from build123d import *

# Parameters (mm, degrees)
F1_DEPTH = 12


with BuildPart() as f1:
    # F0 (on Top) → F1 (new body)
    with BuildSketch(Plane.XY):
        Polygon((395, 100), (0, 100), (-395, 100), (-395, -100), (0, -100), (395, -100), align=None)
        with BuildLine():
            Line((-285.5, 60), (-243.5, 60))
            ThreePointArc((-243.5, 60), (-239.257359, 58.242641), (-237.5, 54))
            Line((-237.5, 54), (-237.5, -54))
            ThreePointArc((-237.5, -54), (-239.257359, -58.242641), (-243.5, -60))
            Line((-243.5, -60), (-285.5, -60))
            ThreePointArc((-285.5, -60), (-289.742641, -58.242641), (-291.5, -54))
            Line((-291.5, -54), (-291.5, 54))
            ThreePointArc((-291.5, 54), (-289.742641, 58.242641), (-285.5, 60))
        make_face(mode=Mode.SUBTRACT)
        with BuildLine():
            ThreePointArc((237.5, 54), (239.257359, 58.242641), (243.5, 60))
            Line((243.5, 60), (285.5, 60))
            ThreePointArc((285.5, 60), (289.742641, 58.242641), (291.5, 54))
            Line((291.5, 54), (291.5, -54))
            ThreePointArc((291.5, -54), (289.742641, -58.242641), (285.5, -60))
            Line((285.5, -60), (243.5, -60))
            ThreePointArc((243.5, -60), (239.257359, -58.242641), (237.5, -54))
            Line((237.5, -54), (237.5, 54))
        make_face(mode=Mode.SUBTRACT)
    extrude(amount=F1_DEPTH)


solid = f1.part
Can you work these out from the model? Positions are in its coordinate system, mm. Round coordinates to 2 decimals unless told otherwise and drop trailing zeros. Write each loop counter-clockwise with the first axis right and the second up, starting at its lowest first coordinate (ties: lowest second). Pieces come first, ordered by that corner, then holes. Notation, with made-up numbers: (-15.75, -12) - (43.25, -12) arc R6 cw to (43.25, -7) - close; hole circle Ø6 at (66, 11). An arc over 180 degrees is marked (long way). Write each question's results on one line, items separated by ' | '. Start each with the question number.
1) Suppose I cut it at C-C (z = 2.5). List the corners of the cut face in (x, y) for me.
2) Please list where these lines run through material, in increasing order: line 1 (X direction, y = 28, z = 2.25); line 2 (Y direction, x = -274.5, z = 4.75); line 3 (X direction, y = -57, z = 6).
3) Suppose I cut it at A-A (x = 267.5). List the corners of the cut face in (y, z) for me, and give its area (3 significant figures).
4) Suppose I cut it at B-B (y = 32.5). List the corners of the cut face in (x, z) for me.
Here are the results:
1) outline: (-395, -100) - (395, -100) - (395, 100) - (-395, 100) - close; hole (-291.5, -54) arc R6 ccw to (-285.5, -60) - (-243.5, -60) arc R6 ccw to (-237.5, -54) - (-237.5, 54) arc R6 ccw to (-243.5, 60) - (-285.5, 60) arc R6 ccw to (-291.5, 54) - close; hole (237.5, -54) arc R6 ccw to (243.5, -60) - (285.5, -60) arc R6 ccw to (291.5, -54) - (291.5, 54) arc R6 ccw to (285.5, 60) - (243.5, 60) arc R6 ccw to (237.5, 54) - close
2) line 1: x = -395 to -291.5, -237.5 to 237.5, 291.5 to 395 | line 2: y = -100 to -60, 60 to 100 | line 3: x = -395 to -290.7, -238.3 to 238.3, 290.7 to 395
3) outline: (-100, 0) - (-60, 0) - (-60, 12) - (-100, 12) - close; (60, 0) - (100, 0) - (100, 12) - (60, 12) - close | area: 960 mm2
4) outline: (-395, 0) - (-291.5, 0) - (-291.5, 12) - (-395, 12) - close; (-237.5, 0) - (237.5, 0) - (237.5, 12) - (-237.5, 12) - close; (291.5, 0) - (395, 0) - (395, 12) - (291.5, 12) - close
